Design review of the part built by this model. Coordinates are the model's own, in mm. Give positions to 0.01 mm unless a question says otherwise; leave off trailing zeros. Use a Markdown table: item, result. Add a question column.
1. To check wall thickness, follow line 1 (X direction, y = 2.7, z = 5); line 2 (Z direction, x = 0, y = 2.7). State the ranges of each line that lie inside material, in increasing order.
2. Add section A-A (z = 4.5). Count the separate pieces of the cut face and the enclosed holes in it, and give its area (3 significant figures).
3. For pin 1 Ø2 at (x, z) = (0, 5) entering from -Y, flat-tipped, find the tip position at first contact; note if it passes through.
4. Draft analysis for pull direction Y (two halves, no side actions). For faces 1 (the flat face through (1, -5, 4)), 2 (the flat face through (-1, 1, 10)), 3 (the cylindrical face through (-1.25, -0.05, 1.26)), 4 (the cylindrical face through (-1.25, -0.05, 8.7)), state which applies: pulls with the +Y half, pulls with the -Y half, needs draft (parallel to the pull), parting line crosses it, or undercut.
Autodesk Fusion 360 part; units mm, degrees
sketch "Sketch1" plane through (0, 0, 0) normal (0, 0, 1) x (1, 0, 0)
  circle A0 centre (0, 0) radius 1.25
  line L0 (5, -5) -> (-5, -5)
  line L1 (-5, -5) -> (-5, 5)
  line L2 (-5, 5) -> (5, 5)
  line L3 (5, 5) -> (5, -5)
  line L4 (5, -5) -> (-5, 5) construction
  line L5 (-5, -5) -> (5, 5) construction
  line L6 (0, -5) -> (0, 5) construction
  line L7 (5, 0) -> (-5, 0) construction
  dimension "d1" = 2.5
  dimension "d3" = 10
  dimension "d4" = 10
ref_plane "WorkPlane1" through (0, -5, 0) normal (0, 1, 0) x (-1, 0, 0)
sketch "Sketch2" plane through (0, -5, 0) normal (0, 1, 0) x (1, 0, 0)
  line L0 (-5, 0) -> (5, 0)
  line L1 (5, 0) -> (5, -10)
  line L2 (5, -10) -> (-5, -10)
  line L3 (-5, -10) -> (-5, 0)
  line L4 (0, 0) -> (0, -10) construction
  circle A0 centre (0, -5) radius 1.25
  point P0 (5, 0)
  point P1 (-5, 0)
  point P2 (5, 0)
  dimension "d6" = 10
  dimension "d8" = 2.5
ref_plane "WorkPlane2" through (-5, 0, 0) normal (1, 0, 0) x (0, 1, 0)
sketch "Sketch3" plane through (-5, 0, 0) normal (1, 0, 0) x (0, 1, 0)
  line L0 (5, 0) -> (-5, 0)
  line L1 (-5, 0) -> (-5, 10)
  line L2 (-5, 10) -> (5, 10)
  line L3 (5, 10) -> (5, 0)
  line L4 (0, 0) -> (0, 10) construction
  circle A0 centre (0, 5) radius 1.25
  point P0 (-5, 0)
  point P1 (-5, 10)
  point P2 (5, 0)
  dimension "d10" = 2.5
ref_plane "WorkPlane3" through (0, 5, 0) normal (0, -1, 0) x (1, 0, 0)
sketch "Sketch4" plane through (0, 5, 0) normal (0, -1, 0) x (1, 0, 0)
  line L0 (5, 0) -> (5, 10)
  line L1 (5, 10) -> (-5, 10)
  circle A0 centre (0, 5) radius 1.25
  line L2 (-5, 0) -> (-5, 10)
  line L3 (-5, 0) -> (5, 0)
ref_plane "WorkPlane4" through (5, 0, 0) normal (-1, 0, 0) x (0, -1, 0)
sketch "Sketch5" plane through (5, 0, 0) normal (-1, 0, 0) x (0, 1, 0)
  line L0 (-5, -10) -> (-5, 0)
  line L1 (-5, -10) -> (5, -10)
  circle A0 centre (0, -5) radius 1.25
  line L2 (5, 0) -> (-5, 0)
  line L3 (5, -10) -> (5, 0)
ref_plane "WorkPlane5" through (0, -5, 10) normal (0, 0, 1) x (-1, 0, 0)
sketch "Sketch6" plane through (0, -5, 10) normal (0, 0, 1) x (1, 0, 0)
  line L0 (-5, 0) -> (5, 0)
  circle A0 centre (0, 5) radius 1.25
  line L1 (-5, 10) -> (5, 10)
  line L2 (-5, 0) -> (-5, 10)
  line L3 (5, 10) -> (5, 0)
ref_plane "WorkPlane6" through (-5, 5, 0) normal (0.5774, -0.5774, -0.5774) x (0.7071, 0.7071, 0)
ref_plane "WorkPlane7" through (-8.3333, 8.3333, 3.3333) normal (0.5774, -0.5774, -0.5774) x (0.7071, 0.7071, 0)
sketch "Sketch7" plane through (-8.3333, 8.3333, 3.3333) normal (0.5774, -0.5774, -0.5774) x (0.7071, 0.7071, 0)
  circle A0 centre (0, 8.165) radius 1.25
  point P0 (0, 8.165)
  point P1 (0, 8.165)
  point P2 (0, 8.165)
  dimension "d25" = 2.5
ref_plane "WorkPlane8" through (-5, -5, 0) normal (0.5774, 0.5774, -0.5774) x (-0.7071, 0.7071, 0)
ref_plane "WorkPlane9" through (-8.3333, -8.3333, 3.3333) normal (0.5774, 0.5774, -0.5774) x (-0.7071, 0.7071, 0)
sketch "Sketch8" plane through (-8.3333, -8.3333, 3.3333) normal (0.5774, 0.5774, -0.5774) x (-0.7071, 0.7071, 0)
  circle A0 centre (0, 8.165) radius 1.25
  point P0 (0, 8.165)
  point P1 (0, 8.165)
  point P2 (0, 8.165)
  dimension "d24" = 2.5
ref_plane "WorkPlane10" through (5, -5, 0) normal (-0.5774, 0.5774, -0.5774) x (-0.7071, -0.7071, 0)
ref_plane "WorkPlane11" through (8.3333, -8.3333, 3.3333) normal (-0.5774, 0.5774, -0.5774) x (-0.7071, -0.7071, 0)
sketch "Sketch9" plane through (8.3333, -8.3333, 3.3333) normal (-0.5774, 0.5774, -0.5774) x (-0.7071, -0.7071, 0)
  circle A0 centre (0, 8.165) radius 1.25
  point P0 (0, 8.165)
  point P1 (0, 8.165)
  point P2 (0, 8.165)
  dimension "d23" = 2.5
ref_plane "WorkPlane12" through (5, 5, 0) normal (-0.5774, -0.5774, -0.5774) x (0.7071, -0.7071, 0)
ref_plane "WorkPlane13" through (8.3333, 8.3333, 3.3333) normal (-0.5774, -0.5774, -0.5774) x (0.7071, -0.7071, 0)
sketch "Sketch10" plane through (8.3333, 8.3333, 3.3333) normal (-0.5774, -0.5774, -0.5774) x (0.7071, -0.7071, 0)
  circle A0 centre (0, 8.165) radius 1.25
  point P0 (0, 8.165)
  point P1 (0, 8.165)
  point P2 (0, 8.165)
  dimension "d22" = 2.5
extrude "Extrude1" add sketch "Sketch1" along normal up to surface (10 mm away) contours A0 | L0 L1 L2 L3
extrude "Extrude2" cut sketch "Sketch3" along normal through all contours A0
extrude "Extrude3" cut sketch "Sketch2" along normal through all contours A0
extrude "Extrude4" cut sketch "Sketch1" along normal through all contours A0
extrude "Extrude5" cut sketch "Sketch10" along normal through all
extrude "Extrude6" cut sketch "Sketch7" along normal through all
extrude "Extrude7" cut sketch "Sketch8" along normal through all
extrude "Extrude8" cut sketch "Sketch9" along normal through all
equation "d1 = TubeDiamter"
equation "TubeDiamter = 2.5 mm"
equation "d3 = CubeSize"
equation "d4 = CubeSize"
equation "d6 = CubeSize"
equation "CubeSize = 10 mm"
equation "d8 = TubeDiamter"
equation "d10 = TubeDiamter"
equation "d22 = TubeDiamter"
equation "d23 = TubeDiamter"
equation "d24 = TubeDiamter"
equation "d25 = TubeDiamter"
Taken from the geometry:
| question | item | result |
|---|---|---|
| 1 | line 1 | x = -5 to -1.25, 1.25 to 5 |
| 1 | line 2 | z = 0 to 3.75, 6.25 to 10 |
| 2 | separate pieces | 4 |
| 2 | enclosed holes | 0 |
| 2 | area | 55.0 mm^2 |
| 3 | pin 1 | passes through |
| 4 | face 1 | pulls with the -Y half |
| 4 | face 2 | needs draft |
| 4 | face 3 | undercut |
| 4 | face 4 | undercut |
